```python
from build123d import *

# Parameters (mm, degrees)
F0_W        = 59.5
F0_H        = 59.5
F1_DEPTH    = 15
F0_W_2      = 63
F0_H_2      = 63
F2_DEPTH    = 4
F3_T1_DEPTH = 87.4948974279
F3_T3_DEPTH = 87.4948974279
F4_C1_SIZE2 = 1.6076951546
F4_C1_SIZE  = 6
F4_C2_SIZE2 = 1.6076951546
F4_C2_SIZE  = 6
F4_C3_SIZE2 = 1.6076951546
F4_C3_SIZE  = 6
F4_C4_SIZE2 = 1.6076951546
F4_C4_SIZE  = 6
F5_R        = 1


# Not quite as in the source:
# - a fillet or chamfer that OpenCascade refuses, or shapes differently, is made with other operations: its cross-section is extruded or revolved along the edge and cut away or added


with BuildPart() as f1:
    # F0 (on Top) → F1 (new body)
    with BuildSketch(Plane.XY):
        Rectangle(F0_W, F0_H)
    extrude(amount=F1_DEPTH)

    # F0 (on Top) → F2 (join)
    with BuildSketch(Plane.XY):
        Rectangle(F0_W_2, F0_H_2)
        Rectangle(F0_W, F0_H, mode=Mode.SUBTRACT)
    extrude(amount=F2_DEPTH)

    # F3: fillet of radius 5 on 4 edges, made by hand

    # F3_s2 → F3_t1 (cut)
    with BuildSketch(Plane.YZ.offset(-43.7474487139)):
        with BuildLine():
            ThreePointArc((-31.5, 4), (-29.7632981746, 1.1270166538), (-26.6010205144, 0))
            Line((-26.6010205144, 0), (-31.5, 0))
            Line((-31.5, 0), (-31.5, 4))
        make_face()
        with BuildLine():
            ThreePointArc((31.5, 4), (29.7632981746, 1.1270166538), (26.6010205144, 0))
            Line((26.6010205144, 0), (31.5, 0))
            Line((31.5, 0), (31.5, 4))
        make_face()
    extrude(amount=F3_T1_DEPTH, mode=Mode.SUBTRACT)

    # F3_s4 → F3_t3 (cut)
    with BuildSketch(Plane.XZ.offset(-43.7474487139)):
        with BuildLine():
            ThreePointArc((31.5, 4), (29.7632981746, 1.1270166538), (26.6010205144, 0))
            Line((26.6010205144, 0), (31.5, 0))
            Line((31.5, 0), (31.5, 4))
        make_face()
        with BuildLine():
            ThreePointArc((-31.5, 4), (-29.7632981746, 1.1270166538), (-26.6010205144, 0))
            Line((-26.6010205144, 0), (-31.5, 0))
            Line((-31.5, 0), (-31.5, 4))
        make_face()
    extrude(amount=F3_T3_DEPTH, mode=Mode.SUBTRACT)

    # F4: chamfer of 6 x 1.6076951546 on 4 edges, made by hand

    # F4_c1
    f4_c1_edges = [f1.edges().sort_by_distance(p)[0] for p in [
        (0, -29.75, 15),
    ]]
    f4_c1_side = f1.faces().sort_by_distance((0, -29.75, 14.9678460969))[0]
    chamfer(f4_c1_edges, length=F4_C1_SIZE, length2=F4_C1_SIZE2, reference=f4_c1_side)

    # F4_c2
    f4_c2_edges = [f1.edges().sort_by_distance(p)[0] for p in [
        (29.75, 0.8038475773, 15),
    ]]
    f4_c2_side = f1.faces().sort_by_distance((29.75, 0.8038475773, 14.9678460969))[0]
    chamfer(f4_c2_edges, length=F4_C2_SIZE, length2=F4_C2_SIZE2, reference=f4_c2_side)

    # F4_c3
    f4_c3_edges = [f1.edges().sort_by_distance(p)[0] for p in [
        (-0.8038475773, 29.75, 15),
    ]]
    f4_c3_side = f1.faces().sort_by_distance((-0.8038475773, 29.75, 14.9678460969))[0]
    chamfer(f4_c3_edges, length=F4_C3_SIZE, length2=F4_C3_SIZE2, reference=f4_c3_side)

    # F4_c4
    f4_c4_edges = [f1.edges().sort_by_distance(p)[0] for p in [
        (-29.75, 0, 15),
    ]]
    f4_c4_side = f1.faces().sort_by_distance((-29.75, 0, 14.9678460969))[0]
    chamfer(f4_c4_edges, length=F4_C4_SIZE, length2=F4_C4_SIZE2, reference=f4_c4_side)

    # F5
    f5_edges = [f1.edges().sort_by_distance(p)[0] for p in [
        (-29.517588, -29.517588, 0.938765),
        (-29.517588, 29.517588, 0.938765),
        (29.517588, 29.517588, 0.938765),
        (29.517588, -29.517588, 0.938765),
    ]]
    fillet(f5_edges, radius=F5_R)


solid = f1.part
```
Part model, mm, in its own coordinate system. A direction names the side the tool comes from. Round coordinates to 2 decimals unless told otherwise and drop trailing zeros. Loops run counter-clockwise (first coordinate to the right, second up) from the corner with the lowest first, then second, coordinate; pieces in that order, holes last.
1. Slice it at A-A (y = -17.5). Give the cut face in (x, z).
Solutions:
outline: (-31.5, 4) arc R5 ccw to (-26.6, 0) - (26.6, 0) arc R5 ccw to (31.5, 4) - (29.75, 4) - (29.75, 9) - (28.14, 15) - (-28.14, 15) - (-29.75, 9) - (-29.75, 4) - close
2. Slice it at C-C (z = 5). Give the cut face in (x, y).
Solutions:
outline: (-29.75, -29.75) - (29.75, -29.75) - (29.75, 29.75) - (-29.75, 29.75) - close
3. 3-axis set-ups, long thin cutter, end or side, ignore diameter. For faces 1 (the face through (0, 29.75, 6)), 2 (the face through (-29.75, 0, 6)), 3 (the face through (0, -29.75, 6)): which of +Z, -Z, +X, -X, +Y, -Y reach the whole face in a straight line?
Solutions:
face 1: +Z, +X, -X, +Y
face 2: +Z, -X, +Y, -Y
face 3: +Z, +X, -X, -Y
4. Slice it at D-D (z = 13.5). Give the cut face in (x, y).
Solutions:
outline: (-28.54, -28.54) - (28.54, -28.54) - (28.54, 28.54) - (-28.54, 28.54) - close
5. Flat gauge pins, fed straight in: pin 1 (1.5 mm diameter, centred on y = 3.5, z = 7, fed in from +X); pin 2 (4 mm diameter, centred on y = -25, z = 4.5, fed in from +X); pin 3 (4 mm diameter, centred on x = -8, z = 5, fed in from -Y); pin 4 (1.5 mm diameter, centred on y = -17, z = 3, fed in from -X). Where does each tip first touch, or does it go through?
Solutions:
pin 1: stops at x = 29.75
pin 2: stops at x = 31.5
pin 3: stops at y = -31.5
pin 4: stops at x = -31.44
6. Drill centre lines: line 1 along X through (y, z) = (-20.5, 5.25); line 2 along Z through (x, y) = (-27, 18.5). Where is each one in solid material? Low to high.
Solutions:
line 1: x = -29.75 to 29.75
line 2: z = 0.02 to 15
